from build123d import *

# Parameters (mm, degrees)
F0_R     = 1.5875
F0_R_2   = 4.0000047
F1_DEPTH = 1.5875


with BuildPart() as f1:
    # F0 (on Right) → F1 (new body, symmetric)
    with BuildSketch(Plane.YZ):
        with BuildLine():
            ThreePointArc((0, 133.35), (-13.4703841816, 127.7703841816), (-19.05, 114.3))
            Line((-19.05, 114.3), (-19.05, -114.3))
            ThreePointArc((-19.05, -114.3), (0, -133.35), (19.05, -114.3))
            Line((19.05, -114.3), (19.05, 114.3))
            ThreePointArc((19.05, 114.3), (13.4703841816, 127.7703841816), (0, 133.35))
        make_face()
        with Locations((-8.128, -114.3)):
            Circle(F0_R, mode=Mode.SUBTRACT)
        with Locations((0, -114.3)):
            Circle(F0_R_2, mode=Mode.SUBTRACT)
        with Locations((8.128, -114.3)):
            Circle(F0_R, mode=Mode.SUBTRACT)
        with Locations((-8.128, 114.3)):
            Circle(F0_R, mode=Mode.SUBTRACT)
        with BuildLine():
            ThreePointArc((4.0000047, 114.3), (-2.8284304481, 111.4715695519), (0, 118.3000047))
            ThreePointArc((0, 118.3000047), (2.8284304481, 117.1284304481), (4.0000047, 114.3))
        make_face(mode=Mode.SUBTRACT)
        with Locations((8.128, 114.3)):
            Circle(F0_R, mode=Mode.SUBTRACT)
    extrude(amount=F1_DEPTH, both=True)


solid = f1.part
Can you work these out from the model? Positions are in its coordinate system, mm. Round coordinates to 2 decimals unless told otherwise and drop trailing zeros. Use CSV: the item, a comma, the result in double quotes. Start each with the question number.
1) We'd pull the mould along X, two halves only. Please class faces 1 (the cylindrical face through (0.022, -0.419, -133.345)), 2 (the flat face through (-1.588, 0, 2)), 3 (the flat face through (1.588, 0, 2)): released by +X, released by -X, zero draft, split by the parting line, or undercut.
2) Please list where these lines run through material, in increasing order: probe 1 along Y at (x, z) = (-0.35, 114.3); probe 2 along Z at (x, y) = (0.95, 0); probe 3 along Z at (x, y) = (-1.25, 8.5). Write a range as [from, to].
3) If we section it at A-A on x = 0.8: Count the separate pieces of the cut face and the enclosed holes in it, plus the area to 3 significant figures.
4) For pin 1 Ø1.9 at (y, z) = (-8.128, -114.3) entering from +X; pin 2 Ø1.5 at (x, y) = (-0.5, 6) entering from +Z, each with a flat end and sliding along its axis, tell me the tip position at first contact or that it passes through.
Geometry results:
1,face 1,"zero draft"
1,face 2,"released by -X"
1,face 3,"released by +X"
2,probe 1,"y = [-19.05, -9.72], [-6.54, -4], [4, 6.54], [9.72, 19.05]"
2,probe 2,"z = [-133.35, -118.3], [-110.3, 110.3], [118.3, 133.35]"
2,probe 3,"z = [-131.35, -115.84], [-112.76, 112.76], [115.84, 131.35]"
3,separate pieces,"1"
3,enclosed holes,"6"
3,area,"9,720 mm2"
4,pin 1,"passes through"
4,pin 2,"stops at z = 132.61"
